```python
from build123d import *

# Parameters (mm, degrees)
SKETCH2_R             = 25
BOSS_EXTRUDE1_DEPTH   = 30
BOSS_EXTRUDE2_DEPTH   = 10
FILLET1_R             = 10
FILLET2_R             = 6
F_1_0MM_DOWEL_HOLE1_D = 24
F_1_0MM_DOWEL_HOLE2_D = 32


with BuildPart() as part:
    # Sketch1 → Revolve1 (revolve)
    with BuildSketch(Plane.XY, mode=Mode.PRIVATE) as revolve1_sk:
        Polygon((0, 0), (37, 0), (25, 45), (0, 45), align=None)
    revolve(revolve1_sk.sketch.rotate(Axis((0, 45, 0), (0, -1, 0)), 90), axis=Axis((0, 45, 0), (0, -1, 0)))



with BuildPart() as body_2:
    # Sketch2 → Boss-Extrude1 (new, symmetric)
    with BuildSketch(Plane.XY):
        with Locations((70, -35)):
            Circle(SKETCH2_R)
    extrude(amount=BOSS_EXTRUDE1_DEPTH, both=True)


with BuildPart() as part_1:
    add(part.part)

    add(body_2.part)  # Boss-Extrude2 merges body 2
    # Sketch3 → Boss-Extrude2 (add, symmetric)
    with BuildSketch(Plane.XY):
        Polygon((22, 0), (22, -35), (54.188700462, -35), (54.188700462, -25), (38.698729811, -25), (32, 0), align=None)
    extrude(amount=BOSS_EXTRUDE2_DEPTH, both=True)

    # Fillet1
    fillet1_edges = [part_1.edges().sort_by_distance(p)[0] for p in [
        (22, -35, 0),
    ]]
    fillet(fillet1_edges, radius=FILLET1_R)

    # Fillet2
    fillet2_edges = [part_1.edges().sort_by_distance(p)[0] for p in [
        (38.698729811, -25, 0),
    ]]
    fillet(fillet2_edges, radius=FILLET2_R)

    # Ø1.0mm Dowel Hole1 (through all)
    with Locations(Plane(origin=(0, 45, 0), x_dir=(1, 0, 0), z_dir=(0, 1, 0))):
        with Locations((0, 0)):
            Hole(F_1_0MM_DOWEL_HOLE1_D / 2)

    # Ø1.0mm Dowel Hole2 (through all)
    with Locations(Plane.XY.offset(30)):
        with Locations((70, -35)):
            Hole(F_1_0MM_DOWEL_HOLE2_D / 2)


solid = part_1.part
```
Verification items for the finished model (mm, model axes). A direction names the side the tool comes from. Coordinates: 2 decimals unless noted, no trailing zeros. Order: outer loops, then holes, each group sorted by start corner. A loop starts at its lowest first (then second) coordinate and runs counter-clockwise, first axis right, second up. Notation, with made-up numbers: (2.25, 77.5) -> (20.25, 77.5) arc R6 cw to (20.25, 87.5) -> close; hole circle Ø11 at (55, 73.5). An arc over 180 degrees is marked (long way). Answer as CSV lines item,"result". Start each with the question number.
1) Cross-section at A-A, the plane z = 0. Record the boundary of the cut face in (x, y), then the cut area to 3 significant figures.
2) Release check for a two-part mould opening along X. For faces 6 (the face through (39.7, -23.8, -0.1)), 7 (the face through (-28.009, 32.815, -3.678)), 8 (the face through (38, -35, 0)), 9 (the face through (11.99, 22.18, -0.53)) record: released by +X, released by -X, zero draft, split by the parting line, or undercut.
3) Gauge pin test, flat ends, axial feed: pin 1 Ø1.9 at (x, z) = (46, -4.5) entering from +Y; pin 2 Ø1 at (y, z) = (23.5, 3.5) entering from -X; pin 3 Ø6 at (y, z) = (31, -29) entering from -X; pin 4 Ø19 at (x, y) = (70, -35) entering from +Z. Record the tip position at first contact, or that the pin passes through.
4) Cross-section at B-B, the plane x = 0. Record the boundary of the cut face in (y, z).
5) Cross-section at D-D, the plane y = -41. Record the boundary of the cut face in (x, z).
6) Cross-section at C-C, the plane y = -27. Record the boundary of the cut face in (x, z).
7) Set-up check for faces 1 (the face through (34.79, -10.42, 0.14)), 2 (the face through (-6, 45, 11)), 3 (the face through (22, -12, 0)), 4 (the face through (45, -25, 0)), 5 (the face through (69.6, -51.3, -30)): record each of +Z, -Z, +X, -X, +Y, -Y from which the full face is reachable in a straight line by a thin tool's end or side.
8) Material ranges on L1, parallel to Y at x = 70, z = -13; L2, parallel to Z at x = 42, y = -33.5; L3, parallel to Z at x = 60, y = -50, recorded low to high. Write a range as [from, to].
Conclusion:
1,outline,"(-37, 0) -> (-12, 0) -> (-12, 45) -> (-25, 45) -> close; (12, 0) -> (22, 0) -> (22, -25) arc R10 ccw to (32, -35) -> (45, -35) arc R25 ccw (long way) to (47.09, -25) -> (43.3, -25) arc R6 cw to (37.51, -20.55) -> (32, 0) -> (37, 0) -> (25, 45) -> (12, 45) -> close; hole circle Ø32 at (70, -35)"
1,area,"3,420 mm²"
2,face 6,"undercut"
2,face 7,"split by the parting line"
2,face 8,"zero draft"
2,face 9,"undercut"
3,pin 1,"stops at y = -25"
3,pin 2,"stops at x = -30.68"
3,pin 3,"stops at x = -12.5"
3,pin 4,"passes through"
4,outline,"(0, -37) -> (45, -25) -> (45, -12) -> (0, -12) -> close; (0, 12) -> (45, 12) -> (45, 25) -> (0, 37) -> close"
5,outline,"(45.73, -30) -> (55.17, -30) -> (55.17, 30) -> (45.73, 30) -> close; (84.83, -30) -> (94.27, -30) -> (94.27, 30) -> (84.83, 30) -> close"
6,outline,"(22.2, -10) -> (46.31, -10) -> (46.31, -30) -> (56.14, -30) -> (56.14, 30) -> (46.31, 30) -> (46.31, 10) -> (22.2, 10) -> close; (83.86, -30) -> (93.69, -30) -> (93.69, 30) -> (83.86, 30) -> close"
7,face 1,"+Z, -Z"
7,face 2,"+Z, -Z, +X, -X, +Y"
7,face 3,"+Z, -Z, -X, -Y"
7,face 4,"+Z, -Z, +Y"
7,face 5,"-Z, +X, -X, +Y, -Y"
8,L1,"y = [-60, -51], [-19, -10]"
8,L2,"z = [-10, 10]"
8,L3,"z = [-30, 30]"
